Job drawing, mm, ordinate dimensions from the low corner. One solid piece. Round coordinates to 2 decimals unless told otherwise and drop trailing zeros. Loops run counter-clockwise (first coordinate to the right, second up) from the corner with the lowest first, then second, coordinate; pieces in that order, holes last.
1) Band-saw the part on D-D, the plane y = 24.9. Write the cut outline in (x, z).
2) Drop flat-ended pins along their axis: P1, Ø4, axis at x = 24.9, y = 6.8, coming from the -Z side; P2, Ø2.5, axis at x = 16.9, y = 34.8, coming from the -Z side. Give the stop position or say it passes through.
3) Band-saw the part on C-C, the plane z = 0.5. State how many separate pieces and enclosed holes the cut face has, then the cut area to 3 significant figures.
4) Band-saw the part on A-A, the plane x = 24.9. Write the cut outline in (y, z).
5) Probe line 1 (Y direction, x = 16.9, z = 0.2); line 2 (Y direction, x = 24.9, z = 0.7); line 3 (X direction, y = 34.8, z = 0.6). List the from-to ranges inside material, lowest first.
6) Band-saw the part on B-B, the plane y = 34.8. Write the cut outline in (x, z).
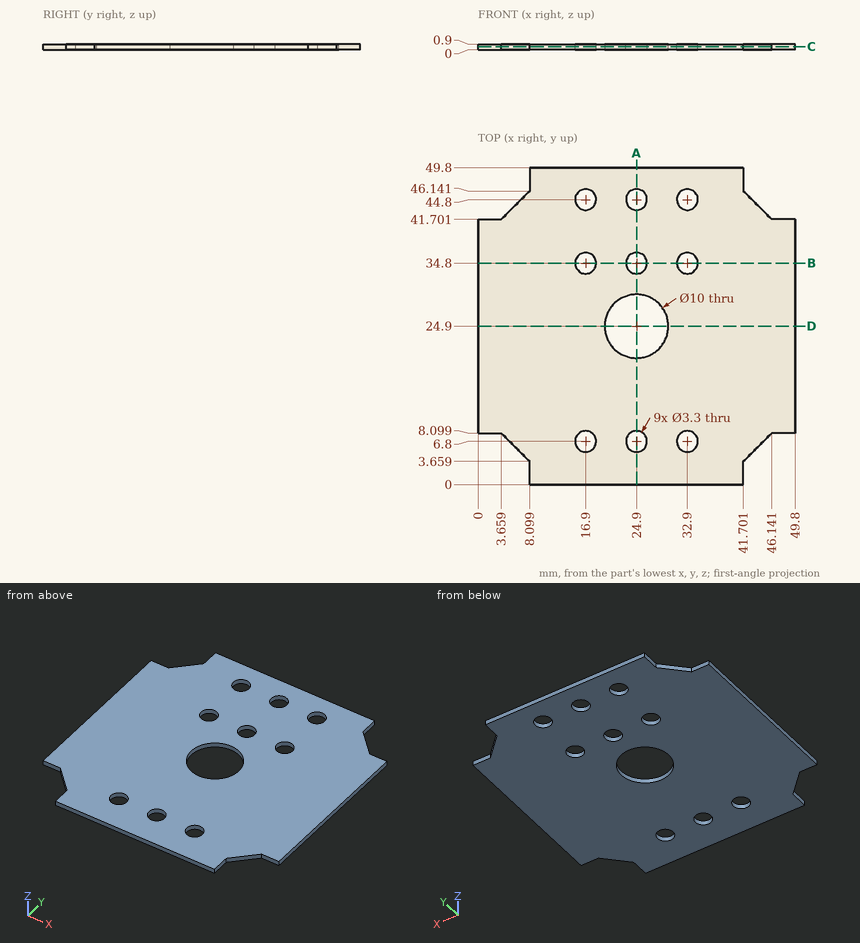
Reported:
1. outline: (0, 0) - (19.9, 0) - (19.9, 0.9) - (0, 0.9) - close; (29.9, 0) - (49.8, 0) - (49.8, 0.9) - (29.9, 0.9) - close
2. P1: stops at z = 0
2. P2: passes through
3. separate pieces: 1
3. enclosed holes: 10
3. area: 2,100 mm2
4. outline: (0, 0) - (5.15, 0) - (5.15, 0.9) - (0, 0.9) - close; (8.45, 0) - (19.9, 0) - (19.9, 0.9) - (8.45, 0.9) - close; (29.9, 0) - (33.15, 0) - (33.15, 0.9) - (29.9, 0.9) - close; (36.45, 0) - (43.15, 0) - (43.15, 0.9) - (36.45, 0.9) - close; (46.45, 0) - (49.8, 0) - (49.8, 0.9) - (46.45, 0.9) - close
5. line 1: y = 0 to 5.15, 8.45 to 33.15, 36.45 to 43.15, 46.45 to 49.8
5. line 2: y = 0 to 5.15, 8.45 to 19.9, 29.9 to 33.15, 36.45 to 43.15, 46.45 to 49.8
5. line 3: x = 0 to 15.25, 18.55 to 23.25, 26.55 to 31.25, 34.55 to 49.8
6. outline: (0, 0) - (15.25, 0) - (15.25, 0.9) - (0, 0.9) - close; (18.55, 0) - (23.25, 0) - (23.25, 0.9) - (18.55, 0.9) - close; (26.55, 0) - (31.25, 0) - (31.25, 0.9) - (26.55, 0.9) - close; (34.55, 0) - (49.8, 0) - (49.8, 0.9) - (34.55, 0.9) - close
